The listing builds one solid part. Answer for the finished solid, in the listing's coordinates (mm). A direction names the side the tool comes from. Coordinates: 2 decimals unless noted, no trailing zeros. Answer as CSV lines item,"result". Start each with the question number.
```python
from build123d import *

# Parameters (mm, degrees)
F1_DEPTH = 4
F3_DEPTH = 4.001
F4_SIZE  = 1.5
F5_R     = 0.5


with BuildPart() as f1:
    # F0 (on Top) → F1 (new body)
    with BuildSketch(Plane.XY):
        with BuildLine():
            Line((-16.7304610461, 10), (-16.7304610461, 0))
            Line((-16.7304610461, 0), (-16.7304610461, -10))
            Line((-16.7304610461, -10), (33.2695389539, -10))
            ThreePointArc((33.2695389539, -10), (43.2695389539, 0), (33.2695389539, 10))
            Line((33.2695389539, 10), (-16.7304610461, 10))
        make_face()
    extrude(amount=F1_DEPTH)

    # F2 (on face) → F3 (cut, through all)
    with BuildSketch(Plane.XY.offset(4)):
        with BuildLine():
            Line((37.6543869574, -0.75), (43.2413742915, -0.75))
            ThreePointArc((43.2413742915, -0.75), (43.2695389539, 0), (43.2413742915, 0.75))
            Line((43.2413742915, 0.75), (37.6543869574, 0.75))
            ThreePointArc((37.6543869574, 0.75), (37.7405832684, 0.3793942482), (37.7695389539, 0))
            ThreePointArc((37.7695389539, 0), (37.7405832684, -0.3793942482), (37.6543869574, -0.75))
        make_face()
        with BuildLine():
            ThreePointArc((37.6543869574, 0.75), (32.7695389539, 0), (37.6543869574, -0.75))
            Line((37.6543869574, -0.75), (35.2695389539, -0.75))
            Line((35.2695389539, -0.75), (35.2695389539, 0.75))
            Line((35.2695389539, 0.75), (37.6543869574, 0.75))
        make_face()
        with BuildLine():
            Line((35.2695389539, -0.75), (37.6543869574, -0.75))
            ThreePointArc((37.6543869574, -0.75), (37.7405832684, -0.3793942482), (37.7695389539, 0))
            ThreePointArc((37.7695389539, 0), (37.7405832684, 0.3793942482), (37.6543869574, 0.75))
            Line((37.6543869574, 0.75), (35.2695389539, 0.75))
            Line((35.2695389539, 0.75), (35.2695389539, -0.75))
        make_face()
    extrude(amount=-F3_DEPTH, mode=Mode.SUBTRACT)

    # F4
    f4_edges = [f1.edges().sort_by_distance(p)[0] for p in [
        (32.769539, 0, 4),
        (32.769539, 0, 0),
    ]]
    chamfer(f4_edges, length=F4_SIZE)

    # F5
    f5_edges = [f1.edges().sort_by_distance(p)[0] for p in [
        (32.769539, 0, 2.5),
        (32.769539, 0, 1.5),
    ]]
    fillet(f5_edges, radius=F5_R)


solid = f1.part
```
1) Find the intervals of material crossed by line 1 (X direction, y = 0, z = 2.1); line 2 (X direction, y = 2, z = 2.2); line 3 (Y direction, x = 33.5, z = 1.3), in increasing order. Write a range as from..to.
2) Which of the six approach directions +Z, -Z, +X, -X, +Y, -Y give full straight-line access (tool end or side, diameter ignored) to faces 4 (the face through (-16.73, 0, 2)), 5 (the face through (40, 0.75, 2))?
3) For a pull along X with two mould halves and no side action, classify faces 1 (the face through (40, -0.75, 2)), 2 (the face through (40.147, 7.26, 1.972)), 3 (the face through (32.41, 0.12, 1.14)) as +X half, -X half, draft (parallel to the pull), parting line (faces both ways), or undercut.
Completed:
1,line 1,"-16.73..32.77"
1,line 2,"-16.73..33.77, 36.77..43.07"
1,line 3,"-10..-2.04, 2.04..10"
2,face 4,"+Z, -Z, -X, +Y, -Y"
2,face 5,"+Z, -Z, +X"
3,face 1,"draft"
3,face 2,"+X half"
3,face 3,"undercut"
